The listing builds one solid part. Answer for the finished solid, in the listing's coordinates (mm). A direction names the side the tool comes from. Round coordinates to 2 decimals unless told otherwise and drop trailing zeros. Write each loop counter-clockwise with the first axis right and the second up, starting at its lowest first coordinate (ties: lowest second). Pieces come first, ordered by that corner, then holes. Notation, with made-up numbers: (36.5, -12.75) - (74.5, -12.75) arc R24 cw to (74.5, 19.25) - close; hole circle Ø11 at (6.25, 56). An arc over 180 degrees is marked (long way). Use a Markdown table: item, result. Add a question column.
1) A cutting plane is placed at B-B (y = 6.5). Give the vertices of the cut face in (x, z), then the cut area to 3 significant figures.
2) Determine the mould class of faces 1 (the flat face through (31, 10.35, 1)), 2 (the cylindrical face through (-2.114, 5.925, 0.986)), 3 (the cylindrical face through (36.85, 6.42, 0.99)) for opening direction Y: +Y half, -Y half, draft (parallel to the pull), parting line (faces both ways), or undercut.
3) A cutting plane is placed at A-A (z = 5). Give the vertices of the cut face in (x, y).
4) A cutting plane is placed at D-D (x = 9). Give the vertices of the cut face in (y, z).
5) A cutting plane is placed at C-C (x = 3.65). Give the vertices of the cut face in (y, z).
6) Each of these flat-tipped pins is pushed along its axis until it touches: P1, Ø1.6, axis at y = 1.5, z = 1, coming from the +X side; P2, Ø0.6, axis at x = 30.5, z = 1.5, coming from the -Y side; P3, Ø3, axis at y = 14.5, z = 7, coming from the -X side; P4, Ø2, axis at y = 1.5, z = 1, coming from the -X side. Where does it stop, or does it pass through?
7) Find the intervals of material crossed by probe 1 along Y at (x, z) = (33, 0.9); probe 2 along Z at (x, y) = (24.35, 17.5); probe 3 along X at (y, z) = (7.5, 0.5), in increasing order. Write a range as from..to.
8) A tool of negligible diameter and unlimited length cuts with its end or side. For faces 4 (the flat face through (15, 16.35, 5)), 5 (the flat face through (0, 17, 3)), 6 (the flat face through (-2, 2.65, 1)), from which of +Z, -Z, +X, -X, +Y, -Y can it reach the whole face along a straight path? Write none if from no direction.
```python
from build123d import *

# Parameters (mm, degrees)
SKETCH1_R           = 1.5
SKETCH1_W           = 25.5
SKETCH1_H           = 14.35
BOSS_EXTRUDE1_DEPTH = 2
SKETCH2_W           = 29.5
SKETCH2_H           = 2
BOSS_EXTRUDE2_DEPTH = 8
SKETCH3_R           = 1.5
CUT_EXTRUDE1_DEPTH  = 8


with BuildPart() as part:
    # Sketch1 → Boss-Extrude1 (new body)
    with BuildSketch(Plane.XY):
        with BuildLine():
            Line((0, 18.35), (0, 10.35))
            Line((0, 10.35), (-3.5, 10.35))
            ThreePointArc((-3.5, 10.35), (-7.35, 6.5), (-3.5, 2.65))
            Line((-3.5, 2.65), (0, 2.65))
            Line((0, 2.65), (0, 0))
            Line((0, 0), (29.5, 0))
            Line((29.5, 0), (29.5, 2.65))
            Line((29.5, 2.65), (33, 2.65))
            ThreePointArc((33, 2.65), (36.85, 6.5), (33, 10.35))
            Line((33, 10.35), (29.5, 10.35))
            Line((29.5, 10.35), (29.5, 18.35))
            Line((29.5, 18.35), (0, 18.35))
        make_face()
        with Locations((-3.5, 6.5)):
            Circle(SKETCH1_R, mode=Mode.SUBTRACT)
        with Locations(Location((33, 6.5, 0), (0, 0, 180))):
            Circle(SKETCH1_R, mode=Mode.SUBTRACT)
        with Locations((14.75, 9.175)):
            Rectangle(SKETCH1_W, SKETCH1_H, mode=Mode.SUBTRACT)
    extrude(amount=BOSS_EXTRUDE1_DEPTH)

    # Sketch2 → Boss-Extrude2 (add)
    with BuildSketch(Plane.XY.offset(2)):
        with Locations((14.75, 17.35)):
            Rectangle(SKETCH2_W, SKETCH2_H)
    extrude(amount=BOSS_EXTRUDE2_DEPTH)

    # Sketch3 → Cut-Extrude1 (cut)
    with BuildSketch(Plane(origin=(0, 18.35, 0), x_dir=(1, 0, 0), z_dir=(0, 1, 0))):
        with Locations(Location((3.65, -5, 0), (0, 0, 180))):
            Circle(SKETCH3_R)
        with Locations(Location((24.35, -5, 0), (0, 0, 180))):
            Circle(SKETCH3_R)
    extrude(amount=-CUT_EXTRUDE1_DEPTH, mode=Mode.SUBTRACT)


solid = part.part
```
Entries:
| question | item | result |
|---|---|---|
| 1 | outline | (-7.35, 0) - (-5, 0) - (-5, 2) - (-7.35, 2) - close; (-2, 0) - (2, 0) - (2, 2) - (-2, 2) - close; (27.5, 0) - (31.5, 0) - (31.5, 2) - (27.5, 2) - close; (34.5, 0) - (36.85, 0) - (36.85, 2) - (34.5, 2) - close |
| 1 | area | 25.4 mm² |
| 2 | face 1 | +Y half |
| 2 | face 2 | undercut |
| 2 | face 3 | parting line |
| 3 | outline | (0, 16.35) - (2.15, 16.35) - (2.15, 18.35) - (0, 18.35) - close; (5.15, 16.35) - (22.85, 16.35) - (22.85, 18.35) - (5.15, 18.35) - close; (25.85, 16.35) - (29.5, 16.35) - (29.5, 18.35) - (25.85, 18.35) - close |
| 4 | outline | (0, 0) - (2, 0) - (2, 2) - (0, 2) - close; (16.35, 0) - (18.35, 0) - (18.35, 10) - (16.35, 10) - close |
| 5 | outline | (0, 0) - (2, 0) - (2, 2) - (0, 2) - close; (16.35, 0) - (18.35, 0) - (18.35, 3.5) - (16.35, 3.5) - close; (16.35, 6.5) - (18.35, 6.5) - (18.35, 10) - (16.35, 10) - close |
| 6 | P1 | stops at x = 29.5 |
| 6 | P2 | stops at y = 2.65 |
| 6 | P3 | passes through |
| 6 | P4 | stops at x = 0 |
| 7 | probe 1 | y = 2.65..5, 8..10.35 |
| 7 | probe 2 | z = 0..3.5, 6.5..10 |
| 7 | probe 3 | x = -7.22..-4.62, -2.38..2, 27.5..31.88, 34.12..36.72 |
| 8 | face 4 | +Z |
| 8 | face 5 | +Z, -Z, -X, +Y |
| 8 | face 6 | +Z, -Z, -X, -Y |
